Autodesk Inventor part; units mm, degrees
ref_plane "YZ Plane" through (0, 0, 0) normal (1, 0, 0) x (0, 1, 0)
ref_plane "XZ Plane" through (0, 0, 0) normal (0, 1, 0) x (-1, 0, 0)
ref_plane "XY Plane" through (0, 0, 0) normal (0, 0, 1) x (1, 0, 0)
sketch "Schizzo1" plane through (0, 0, 0) normal (0, 0, 1) x (1, 0, 0)
  line L0 (9, 6) -> (9, -6)
  line L1 (6, -9) -> (-6, -9)
  line L2 (-9, -6) -> (-9, 6)
  line L3 (-6, 9) -> (6, 9)
  arc A0 (-6, 9) -> (-9, 6) centre (-6, 6) ccw
  arc A1 (-9, -6) -> (-6, -9) centre (-6, -6) ccw
  arc A2 (6, -9) -> (9, -6) centre (6, -6) ccw
  arc A3 (9, 6) -> (6, 9) centre (6, 6) ccw
  point P0 (0, 0)
  point P1 (0, 0)
  point P2 (9, 9)
  point P3 (9, -9)
  point P4 (-9, -9)
  point P5 (-9, 9)
  dimension "d0" = 18
  dimension "d72" = 3
extrude "Estrusione1" add sketch "Schizzo1" against normal blind 40
sketch "Schizzo2" plane through (0, 0, 0) normal (0, 0, 1) x (1, 0, 0)
  line L0 (24.2, -31.25) -> (-24.2, -31.25)
  line L1 (-24.2, -31.25) -> (-24.2, 31.25)
  line L2 (-24.2, 31.25) -> (24.2, 31.25)
  line L3 (24.2, 31.25) -> (24.2, -31.25)
  line L4 (24.2, -31.25) -> (-24.2, 31.25) construction
  line L5 (-24.2, -31.25) -> (24.2, 31.25) construction
  point P0 (0, 0)
  dimension "d3" = 62.5
  dimension "d4" = 48.4
extrude "Estrusione2" add sketch "Schizzo2" along normal blind 53
sketch "Schizzo3" plane through (-24.2, 31.25, 0) normal (0, 1, 0) x (1, 0, 0)
  line L0 (24.2, 0) -> (24.2, -28.2)
  line L1 (24.2, 0) -> (52.4, 0) construction
  circle A0 centre (24.2, -28.2) radius 18.75
  dimension "d7" = 28.2
  dimension "d8" = 90
  dimension "d9" = 37.5
extrude "Estrusione3" cut sketch "Schizzo3" against normal blind 55.5
sketch "Schizzo14" plane through (0, 0, 0) normal (0, 0, -1) x (-1, 0, 0)
  line L0 (-11, 13) -> (11, 13)
  line L1 (13, 11) -> (13, -11)
  line L2 (11, -13) -> (-11, -13)
  line L3 (-13, -11) -> (-13, 11)
  arc A0 (11, -13) -> (13, -11) centre (11, -11) ccw
  arc A1 (-13, -11) -> (-11, -13) centre (-11, -11) ccw
  arc A2 (13, 11) -> (11, 13) centre (11, 11) ccw
  arc A3 (-11, 13) -> (-13, 11) centre (-11, 11) ccw
  line L4 (-9.382, 10.5) -> (9.382, 10.5)
  line L5 (10.5, 9.382) -> (10.5, -9.382)
  line L6 (9.382, -10.5) -> (-9.382, -10.5)
  line L7 (-10.5, -9.382) -> (-10.5, 9.382)
  arc A4 (-10.1273, 10.8333) -> (-10.8333, 10.1273) centre (-10.5, 10.5) ccw
  arc A5 (-10.1273, 10.8333) -> (-9.382, 10.5) centre (-9.382, 11.5) ccw
  arc A6 (-10.5, 9.382) -> (-10.8333, 10.1273) centre (-11.5, 9.382) ccw
  arc A7 (10.8333, 10.1273) -> (10.1273, 10.8333) centre (10.5, 10.5) ccw
  arc A8 (9.382, 10.5) -> (10.1273, 10.8333) centre (9.382, 11.5) ccw
  arc A9 (10.8333, 10.1273) -> (10.5, 9.382) centre (11.5, 9.382) ccw
  arc A10 (10.1273, -10.8333) -> (10.8333, -10.1273) centre (10.5, -10.5) ccw
  arc A11 (10.1273, -10.8333) -> (9.382, -10.5) centre (9.382, -11.5) ccw
  arc A12 (10.5, -9.382) -> (10.8333, -10.1273) centre (11.5, -9.382) ccw
  arc A13 (-10.8333, -10.1273) -> (-10.1273, -10.8333) centre (-10.5, -10.5) ccw
  arc A14 (-9.382, -10.5) -> (-10.1273, -10.8333) centre (-9.382, -11.5) ccw
  arc A15 (-10.8333, -10.1273) -> (-10.5, -9.382) centre (-11.5, -9.382) ccw
  point P0 (0, 0)
  point P1 (0, 0)
  point P2 (-10.5, 10.5)
  point P3 (10.5, 10.5)
  point P4 (10.5, -10.5)
  point P5 (-10.5, -10.5)
  point P6 (0, 0)
  point P7 (-13, 13)
  point P8 (13, 13)
  point P9 (13, -13)
  point P10 (-13, -13)
  point P11 (0, 0)
  point P12 (-10, 10.5)
  point P13 (-10.5, 10)
  point P14 (10.5, 10)
  point P15 (10, 10.5)
  point P16 (10, -10.5)
  point P17 (10.5, -10)
  point P18 (-10.5, -10)
  point P19 (-10, -10.5)
  dimension "d77" = 21
  dimension "d78" = 26
  dimension "d102" = 2
  dimension "d110" = 1
  dimension "d112" = 1
  dimension "d114" = 1
  dimension "d116" = 1
extrude "Estrusione10" add sketch "Schizzo14" along normal blind 40
sketch "Schizzo15" plane through (-13, 13, 0) normal (0, 1, 0) x (1, 0, 0)
  line L0 (13, 0) -> (13, 13)
  line L1 (13, 0) -> (26, 0) construction
  dimension "d82" = 13
  dimension "d83" = 90
hole "Foro4" at (0, 13, -13) direction (0, -1, 0) diameter 5.5 depth 26
sketch "Schizzo16" plane through (13, -11, 0) normal (1, 0, 0) x (0, 0, -1)
  line L0 (0, 11) -> (27, 11)
  line L1 (0, 11) -> (27, 11) construction
  dimension "d91" = 27
  dimension "d92" = 0
hole "Foro5" at (13, 0, -27) direction (-1, 0, 0) diameter 5.5 depth 26
fillet "Raccordo1" radius 2 1 edges at (0, -13, -40)
fillet "Raccordo2" radius 2 1 edges at (-9, 0, -40)
fillet "Raccordo3" radius 8 1 edges at (-13, 0, 0)
sketch "Schizzo26" plane through (-24.2, -31.25, 0) normal (0, -1, 0) x (1, 0, 0)
  circle A0 centre (24.2, 28.2) radius 18.75
  line L0 (24.2, 46.95) -> (24.2, 27.55)
  line L1 (24.2, 46.95) -> (43.6, 46.95) construction
  line L2 (24.2, 27.55) -> (24.2, 21.55)
  circle A1 centre (24.2, 21.55) radius 6.4
  point P0 (24.2, 0)
  dimension "d159" = 19.4
  dimension "d160" = 90
  dimension "d161" = 6
  dimension "d162" = 180
  dimension "d163" = 12.8
extrude "Estrusione16" cut sketch "Schizzo26" against normal blind 10 contours A1
sketch "Schizzo27" plane through (-24.2, -31.25, 0) normal (0, -1, 0) x (1, 0, 0)
  circle A0 centre (24.2, 28.2) radius 18.75
  line L0 (24.2, 28.2) -> (39.5, 28.2)
  point P0 (24.2, 0)
  point P1 (31.85, 41.4502)
  point P2 (16.55, 41.4502)
  point P3 (8.9, 28.2)
  point P4 (16.55, 14.9498)
  point P5 (31.85, 14.9498)
  dimension "d166" = 15.3
  dimension "d169" = 360
hole "Foro9" at (-15.3, -31.25, 28.2) at (-7.65, -31.25, 41.4502) at (7.65, -31.25, 41.4502) at (15.3, -31.25, 28.2) direction (0, 1, 0) diameter 3.8 depth 8.8 tip angle 118
sketch "Schizzo28" plane through (-24.2, -31.25, 0) normal (-1, 0, 0) x (0, 0, 1)
  line L0 (53, 62.5) -> (53, 0)
  line L1 (53, 0) -> (53, 7)
  line L2 (53, 0) -> (60, 0) construction
  line L3 (53, 7) -> (53, 12)
  line L4 (53, 7) -> (53, 12)
  line L5 (53, 12) -> (37, 12)
  line L6 (53, 12) -> (49.5, 12)
  line L7 (53, 12) -> (56.5, 12) construction
  line L8 (53, 12) -> (49, 12)
  line L9 (37, 12) -> (37, 7)
  line L10 (37, 12) -> (42, 12) construction
  line L11 (37, 7) -> (49, 7)
  line L12 (49, 7) -> (49, 12)
  line L13 (49, 12) -> (37, 12)
  line L14 (37, 12) -> (37, 7)
  line L15 (53, 62.5) -> (53, 53.5)
  line L16 (53, 62.5) -> (62, 62.5) construction
  line L17 (53, 62.5) -> (53, 53.5)
  line L18 (53, 53.5) -> (37, 53.5)
  line L19 (37, 53.5) -> (37, 62.5)
  line L20 (37, 62.5) -> (53, 62.5)
  point P0 (0, 31.25)
  dimension "d178" = 7
  dimension "d179" = 90
  dimension "d180" = 5
  dimension "d181" = 180
  dimension "d184" = 180
  dimension "d185" = 4
  dimension "d186" = 5
  dimension "d187" = 90
  dimension "d188" = 9
  dimension "d189" = 90
  dimension "d190" = 16
extrude "Estrusione17" cut sketch "Schizzo28" against normal through all
full round fillet "Raccordo5" first side at (24.2, -6.4167, 12.3333) centre faces at (8.0667, -13.4167, 53) second side at (-24.2, -6.4167, 12.3333)
sketch "Schizzo30" plane through (16.5566, 22.25, 37) normal (0, 0, 1) x (1, 0, 0)
  line L0 (-39.325, 9) -> (-33.1133, 9)
  line L1 (0, 9) -> (6.2118, 9)
  line L2 (0, -46.5) -> (0, -41.5)
  line L3 (-33.1133, -41.5) -> (-33.1133, -46.5)
  line L4 (-40.7566, 9) -> (-40.7566, -53.5)
  line L5 (6.2118, 9) -> (6.2118, 0)
  line L6 (7.6434, -53.5) -> (7.6434, 9)
  line L7 (-40.7566, 9) -> (7.6434, 9)
  line L8 (7.6434, 9) -> (7.6434, -46.5)
  line L9 (7.6434, -46.5) -> (-40.7566, -46.5)
  line L10 (-40.7566, -46.5) -> (-40.7566, 9)
  point P0 (-16.5566, -22.25)
  point P1 (-40.7566, -46.5)
  point P2 (7.6434, 9)
  point P3 (-33.1133, 9)
extrude "Estrusione19" cut sketch "Schizzo30" along normal blind 20 and the other way blind 10
sketch "Schizzo31" plane through (0, 0, 0) normal (0, 0, -1) x (-1, 0, 0)
  line L0 (24.2, 31.25) -> (24.2, -31.25)
  line L1 (-24.2, -26.25) -> (24.2, -26.25)
  line L2 (24.2, -26.25) -> (24.2, 26.25)
  line L3 (24.2, 26.25) -> (-24.2, 26.25)
  line L4 (-24.2, 26.25) -> (-24.2, -26.25)
  point P0 (0, 0)
  point P1 (24.2, -26.25)
extrude "Estrusione20" cut sketch "Schizzo31" along normal up to surface (40 mm away)
sketch "Schizzo32" plane through (-24.2, -31.25, 0) normal (0, -1, 0) x (1, 0, 0)
  line L0 (24.2, 0) -> (24.2, -50)
  line L1 (24.2, -50) -> (-25.8, -50)
  line L2 (24.2, -50) -> (74.2, -50)
  line L3 (39.2, 0) -> (9.2, 0)
  line L4 (0, 0) -> (48.4, 0)
  line L5 (-25.8, -50) -> (-25.8, -40)
  line L6 (74.2, -50) -> (-25.8, -50)
  line L7 (-25.8, -50) -> (-25.8, -40)
  line L8 (59.2, -40) -> (74.2, -40)
  line L9 (74.2, -40) -> (74.2, -50)
  line L10 (9.2, -5) -> (9.2, -20)
  line L11 (39.2, -5) -> (39.2, -20)
  arc A0 (39.2, -20) -> (59.2, -40) centre (59.2, -20) ccw
  line L12 (-10.8, -40) -> (-25.8, -40)
  arc A1 (-10.8, -40) -> (9.2, -20) centre (-10.8, -20) ccw
  line L13 (4.2, 0) -> (0, 0)
  line L14 (48.4, 0) -> (48.4, 28.8)
  line L15 (48.4, 0) -> (44.2, 0)
  arc A2 (44.2, 0) -> (39.2, -5) centre (44.2, -5) ccw
  arc A3 (9.2, -5) -> (4.2, 0) centre (4.2, -5) ccw
  point P0 (24.2, 0)
  point P1 (9.2, -40)
  point P2 (9.2, 0)
  point P3 (4.2, 0)
  dimension "d205" = 50
  dimension "d206" = 50
  dimension "d207" = 50
  dimension "d208" = 30
  dimension "d209" = 10
  dimension "d210" = 20
  dimension "d211" = 20
  dimension "d212" = 5
  dimension "d213" = 5
extrude "Estrusione21" add sketch "Schizzo32" against normal blind 40
fillet "Raccordo6" radius 5 1 edges at (0, 8.75, 0)
properties part number "5_Connettore_sup_inf" material "PLA(Stampato)"
Read the model definition and answer for the solid it produces. Units are mm, in the model's axes. A direction names the side the tool comes from. Round coordinates to 2 decimals unless told otherwise and drop trailing zeros. Loops run counter-clockwise (first coordinate to the right, second up) from the corner with the lowest first, then second, coordinate; pieces in that order, holes last.
Q1. Section C-C on y = 23.5 is taken. Write down the section's boundary in (x, z), and give its area (3 significant figures).
Q2. Section D-D on z = -43 is taken. Write down the section's boundary in (x, y), and give its area (3 significant figures).
Q3. Which of the six approach directions +Z, -Z, +X, -X, +Y, -Y give full straight-line access (tool end or side, diameter ignored) to faces 5 (the face through (-16, -9, -2)), 6 (the face through (0, 14, 0)), 7 (the face through (-21, 4, 27)), 8 (the face through (42, -12, -40)), 9 (the face through (-1, 8.75, -32))?
Q4. Section A-A on x = 0 is taken. Write down the section's boundary in (y, z).
Q5. Determine the mould class of faces 1 (the face through (-42, -12, -40)), 2 (the face through (20.703, -11.53, -33.986)), 3 (the face through (0, -24.25, 31)), 4 (the face through (15, -12, -12)) for opening direction Z: released by +Z, released by -Z, zero draft, split by the parting line, or undercut.
Q6. Consider probe 1 along Z at (x, y) = (0, -29); probe 2 along X at (y, z) = (-27, 21); probe 3 along Z at (x, y) = (-45.5, -16). Determine where each line is inside the solid, lowest interval first.
Q7. Section B-B on z = 21.55 is taken. Write down the section's boundary in (x, y).
Q8. Each of these flat-tipped pins is pushed along its axis until it touches: pin 1 (16.5 mm diameter, centred on x = 0, z = 21.55, fed in from +Y); pin 2 (8 mm diameter, centred on x = -25, z = 16, fed in from -Y); pin 3 (1 mm diameter, centred on x = 2.5, y = -20, fed in from +Z); pin 4 (3 mm diameter, centred on x = 3.5, z = -11.5, fed in from +Y). Where does it stop, or does it pass through?
Output:
1. outline: (-24.2, 0) - (24.2, 0) - (24.2, 27) - (18.71, 27) arc R18.75 cw to (-18.71, 27) - (-24.2, 27) - close
1. area: 800 mm2
2. outline: (-50, -31.25) - (50, -31.25) - (50, 8.75) - (-50, 8.75) - close
2. area: 4,000 mm2
3. face 5: -X, +Y, -Y
3. face 6: +Y
3. face 7: +Z, +X, -X, +Y
3. face 8: +Z, +X, +Y, -Y
3. face 9: -Z, +X, -X, +Y
4. outline: (-31.25, -50) - (8.75, -50) - (8.75, -5) arc R5 cw to (13.75, 0) - (31.25, 0) - (31.25, 9.45) - (-24.25, 9.45) - (-24.25, 15.15) - (-31.25, 15.15) - close; (-31.25, 27.95) - (-24.25, 27.95) - (-24.25, 53) - (-31.25, 53) - close
5. face 1: released by +Z
5. face 2: undercut
5. face 3: zero draft
5. face 4: undercut
6. probe 1: z = -50 to 15.15, 27.95 to 53
6. probe 2: x = -24.2 to -6.38, 6.38 to 24.2
6. probe 3: z = -50 to -40
7. outline: (-24.2, -31.25) - (-6.4, -31.25) - (-6.4, -24.25) - (-17.53, -24.25) - (-17.53, 31.25) - (-24.2, 31.25) - close; (6.4, -31.25) - (24.2, -31.25) - (24.2, 31.25) - (17.53, 31.25) - (17.53, -24.25) - (6.4, -24.25) - close
8. pin 1: stops at y = -24.25
8. pin 2: stops at y = -31.25
8. pin 3: stops at z = 9.69
8. pin 4: stops at y = 8.75
